```python
from build123d import *

# Parameters (mm, degrees)
SKETCH1_W            = 81
SKETCH1_H            = 150
BOSS_EXTRUDE1_DEPTH  = 3
M3_CLEARANCE_HOLE1_D = 3.2
SKETCH9_R            = 5.75
SKETCH9_W            = 22
SKETCH9_H            = 27
SKETCH9_W_2          = 11
CUT_EXTRUDE1_DEPTH   = 4


with BuildPart() as part:
    # Sketch1 → Boss-Extrude1 (new body)
    with BuildSketch(Plane(origin=(0, 0, 0), x_dir=(1, 0, 0), z_dir=(0, 1, 0))):
        with Locations((40.5, 75)):
            Rectangle(SKETCH1_W, SKETCH1_H)
    extrude(amount=BOSS_EXTRUDE1_DEPTH)

    # M3 Clearance Hole1 (through all)
    with Locations(Plane(origin=(3, 3, -147), x_dir=(0, 0, 1), z_dir=(0, 1, 0))):
        with Locations((0, 0), (0, 75), (144, 75), (144, 0)):
            Hole(M3_CLEARANCE_HOLE1_D / 2)

    # Sketch9 → Cut-Extrude1 (cut, through all)
    with BuildSketch(Plane(origin=(0, 3, 0), x_dir=(1, 0, 0), z_dir=(0, 1, 0))):
        with Locations((40.5, 25)):
            Circle(SKETCH9_R)
        with Locations((40.5, 125)):
            Rectangle(SKETCH9_W, SKETCH9_H)
        with Locations((40.5, 90)):
            Rectangle(SKETCH9_W, SKETCH9_H)
        with Locations((40.5, 55)):
            Rectangle(SKETCH9_W_2, SKETCH9_H)
    extrude(amount=-CUT_EXTRUDE1_DEPTH, mode=Mode.SUBTRACT)


solid = part.part
```
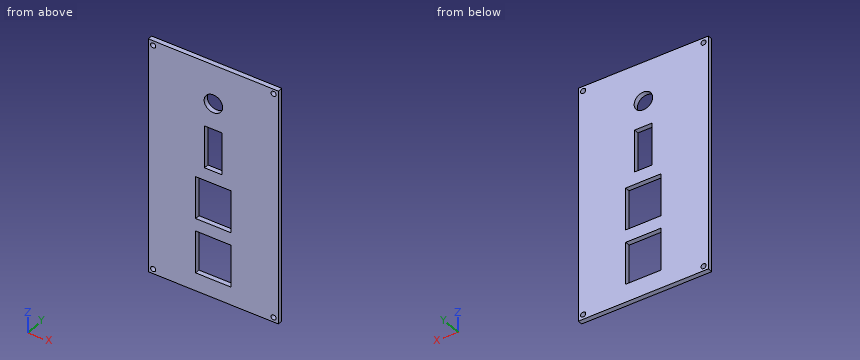
The model under review builds one solid part; all positions refer to its coordinate system, in mm. Round coordinates to 2 decimals unless told otherwise and drop trailing zeros. Write each loop counter-clockwise with the first axis right and the second up, starting at its lowest first coordinate (ties: lowest second). Pieces come first, ordered by that corner, then holes.
(1) Wall thickness on L1, parallel to Z at x = 78, y = 1.55; L2, parallel to X at y = 1.5, z = -147; L3, parallel to X at y = 2.6, z = -119: over which ranges is each line inside the solid? List them lowest first.
(2) We need section D-D on y = 0.6. Give the number of separate pieces and of enclosed holes in the cut face, and give its area (3 significant figures).
(3) We need section B-B on z = -147. Give the boundary of the cut face in (x, y), and give its area (3 significant figures).
(4) We need section A-A on x = 49.5. Give the boundary of the cut face in (y, z).
(5) We need section C-C on z = -57.5. Give the boundary of the cut face in (x, y).
(6) Insertion check: pin 1 (1.5 mm diameter, centred on x = 39.5, y = 1, fed in from +Z); pin 2 (2.5 mm diameter, centred on x = 3, z = -147, fed in from +Y). Each pin has a flat end and moves straight along its axis. Give the tip position at first contact, or say it passes through.
Findings below:
1. L1: z = -150 to -148.6, -145.4 to -4.6, -1.4 to 0
1. L2: x = 0 to 1.4, 4.6 to 76.4, 79.6 to 81
1. L3: x = 0 to 29.5, 51.5 to 81
2. separate pieces: 1
2. enclosed holes: 8
2. area: 10,500 mm2
3. outline: (0, 0) - (1.4, 0) - (1.4, 3) - (0, 3) - close; (4.6, 0) - (76.4, 0) - (76.4, 3) - (4.6, 3) - close; (79.6, 0) - (81, 0) - (81, 3) - (79.6, 3) - close
3. area: 224 mm2
4. outline: (0, -150) - (3, -150) - (3, -138.5) - (0, -138.5) - close; (0, -111.5) - (3, -111.5) - (3, -103.5) - (0, -103.5) - close; (0, -76.5) - (3, -76.5) - (3, 0) - (0, 0) - close
5. outline: (0, 0) - (35, 0) - (35, 3) - (0, 3) - close; (46, 0) - (81, 0) - (81, 3) - (46, 3) - close
6. pin 1: stops at z = 0
6. pin 2: passes through
